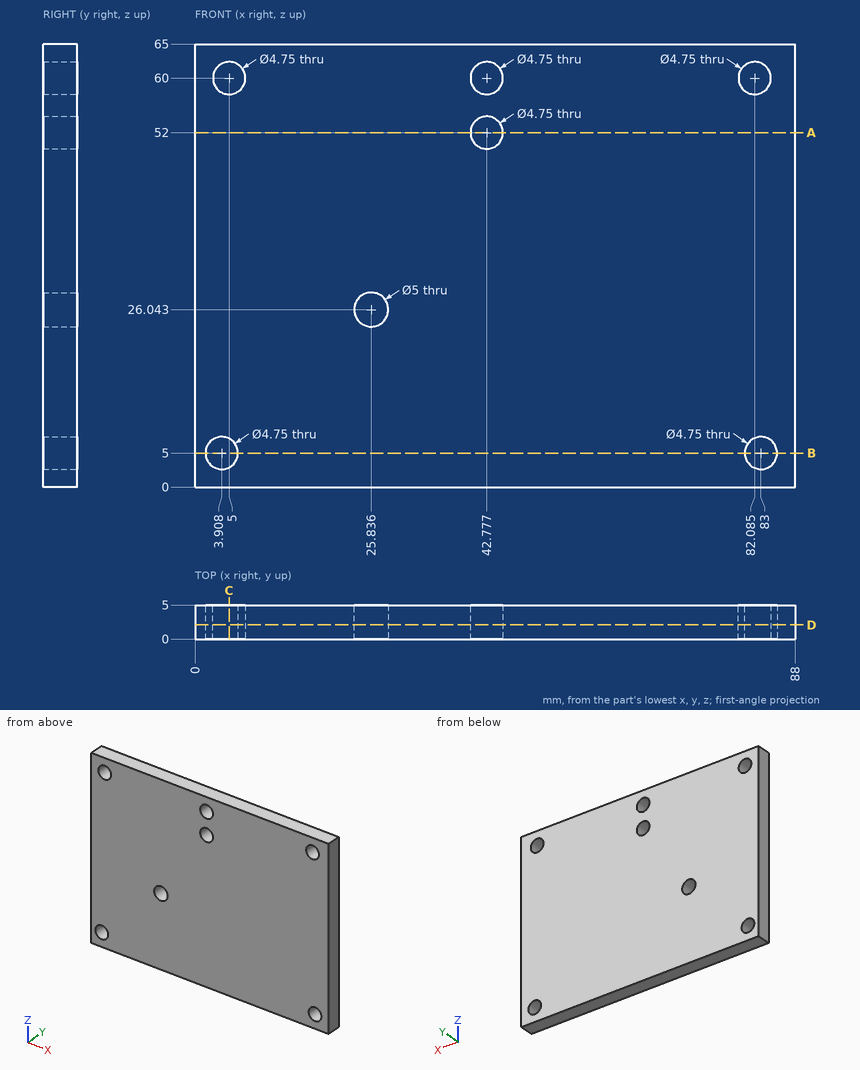
For this review, use the dimensioned drawing (mm, ordinates from the lowest corner) and the shaded views. Round coordinates to 2 decimals unless told otherwise and drop trailing zeros. Order: outer loops, then holes, each group sorted by start corner. A loop starts at its lowest first (then second) coordinate and runs counter-clockwise, first axis right, second up. Notation, with made-up numbers: (-14.5, 30.5) -> (40.5, 30.5) arc R9 ccw to (40.5, 41.5) -> close; hole circle Ø7 at (73, -32). An arc over 180 degrees is marked (long way). One line per item, written item: value. Start each with the question number.
Q1. Take a section at A-A (z = 52). Write out the cut boundary in (x, y), and give its area (3 significant figures).
Q2. Take a section at C-C (x = 5). Write out the cut boundary in (y, z) (1 decimal).
Q3. Wall thickness on line 1 (X direction, y = 1.3, z = 4) (1 decimal); line 2 (X direction, y = 0.6, z = 60.5) (1 decimal); line 3 (Z direction, x = 5, y = 2.2) (1 decimal): over which ranges is each line inside the solid? List them lowest first.
Q4. Take a section at D-D (y = 2.1). Count the separate pieces of the cut face and the enclosed holes in it, and give its area (3 significant figures).
Q5. Take a section at B-B (z = 5). Write out the cut boundary in (x, y) (1 decimal).
Reported:
1. outline: (0, 0) -> (40.4, 0) -> (40.4, 5) -> (0, 5) -> close; (45.15, 0) -> (88, 0) -> (88, 5) -> (45.15, 5) -> close
1. area: 416 mm2
2. outline: (0, 0) -> (5, 0) -> (5, 2.9) -> (0, 2.9) -> close; (0, 7.1) -> (5, 7.1) -> (5, 57.6) -> (0, 57.6) -> close; (0, 62.4) -> (5, 62.4) -> (5, 65) -> (0, 65) -> close
3. line 1: x = 0 to 1.8, 6.1 to 80.8, 85.2 to 88
3. line 2: x = 0 to 2.7, 7.3 to 40.5, 45.1 to 79.8, 84.4 to 88
3. line 3: z = 0 to 2.9, 7.1 to 57.6, 62.4 to 65
4. separate pieces: 1
4. enclosed holes: 7
4. area: 5,590 mm2
5. outline: (0, 0) -> (1.5, 0) -> (1.5, 5) -> (0, 5) -> close; (6.3, 0) -> (80.6, 0) -> (80.6, 5) -> (6.3, 5) -> close; (85.4, 0) -> (88, 0) -> (88, 5) -> (85.4, 5) -> close
